Read the model definition and answer for the solid it produces. Units are mm, in the model's axes. Give positions to 0.01 mm unless a question says otherwise; leave off trailing zeros. Order: outer loops, then holes, each group sorted by start corner. A loop starts at its lowest first (then second) coordinate and runs counter-clockwise, first axis right, second up. Notation, with made-up numbers: (-30.5, 3.5) - (-19.5, 3.5) arc R29 cw to (-19.5, 36.5) - close; hole circle Ø8 at (83, 54). An arc over 180 degrees is marked (long way). Write each question's results on one line, items separated by ' | '.
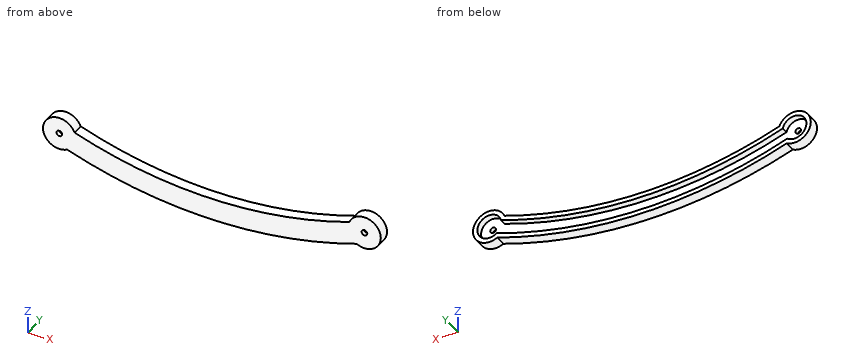
from build123d import *

# Parameters (mm, degrees)
DODANIE_WYCI_GNI_CIE2_DEPTH  = 5
SKORUPA2_START               = 2
SKORUPA2_DEPTH               = 3
SZKIC5_W                     = 1.3
SZKIC5_H                     = 2.001
OTW_R_POD_RUB_M22_AT_2_COUNT = 2
OTW_R_POD_RUB_M22_AT_2_PITCH = 140


# Read off the part's stored shape, not the designer's step: Skorupa2
with BuildPart() as part:
    # Szkic4 → Dodanie-wyciągnięcie2 (new body)
    with BuildSketch(Plane(origin=(0, 0, 0), x_dir=(1, 0, 0), z_dir=(0, 1, 0))):
        with BuildLine():
            ThreePointArc((3.578481933, 6.591241693), (-7.061624869, -2.526549863), (6.947544161, -2.825177894))
            ThreePointArc((6.947544161, -2.825177894), (70, 7.650060048), (133.052455839, -2.825177894))
            ThreePointArc((133.052455839, -2.825177894), (147.061624869, -2.526549863), (136.421518067, 6.591241693))
            ThreePointArc((136.421518067, 6.591241693), (70, 17.650060048), (3.578481933, 6.591241693))
        make_face()
    extrude(amount=DODANIE_WYCI_GNI_CIE2_DEPTH)

    # Skorupa2 outline → Skorupa2 (cut)
    with BuildSketch(Plane(origin=(0, 0, 0), x_dir=(1, 0, 0), z_dir=(0, 1, 0)).offset(SKORUPA2_START)):
        with BuildLine():
            ThreePointArc((3.318777837, 4.385853813), (-5.173966338, -1.865495198), (5.353998671, -1.258847978))
            ThreePointArc((5.353998671, -1.258847978), (70, 9.650060048), (134.646001329, -1.258847978))
            ThreePointArc((134.646001329, -1.258847978), (145.173966338, -1.865495198), (136.681222163, 4.385853813))
            ThreePointArc((136.681222163, 4.385853813), (70, 15.650060048), (3.318777837, 4.385853813))
        make_face()
    extrude(amount=SKORUPA2_DEPTH, mode=Mode.SUBTRACT)

    # Szkic5 → Otwór pod śrubę M22 (revolve, cut)
    with BuildSketch(Plane(origin=(0, 2, 0), x_dir=(0, 0, 1), z_dir=(1, 0, 0))):
        with Locations((0.65, 1.0005)):
            Rectangle(SZKIC5_W, SZKIC5_H)
    otw_r_pod_rub_m22 = revolve(axis=Axis((0, 8.35, 0), (0, -1, 0)), mode=Mode.SUBTRACT)

    # Otwór pod śrubę M22 at 2: Otwór pod śrubę M22 ×2
    with Locations(*[(i * OTW_R_POD_RUB_M22_AT_2_PITCH, 0, 0) for i in range(1, OTW_R_POD_RUB_M22_AT_2_COUNT)]):
        add(otw_r_pod_rub_m22, mode=Mode.SUBTRACT)


solid = part.part
(1) Section B-B (y = 3.7) is taken. Give the vertices of the cut face in (x, z), plus the area to 3 significant figures.
Conclusion:
outline: (3.58, -6.59) arc R205 ccw to (136.42, -6.59) arc R7.5 ccw (long way) to (133.05, 2.83) arc R195 cw to (6.95, 2.83) arc R7.5 ccw (long way) to start; hole (3.32, -4.39) arc R203 ccw to (136.68, -4.39) arc R5.5 ccw (long way) to (134.65, 1.26) arc R197 cw to (5.35, 1.26) arc R5.5 ccw (long way) to start | area: 660 mm^2
(2) Section A-A (x = 140) is taken. Give the vertices of the cut face in (y, z), plus the area to 3 significant figures.
Conclusion:
outline: (0, -7.5) - (5, -7.5) - (5, -5.5) - (2, -5.5) - (2, -1.3) - (0, -1.3) - close; (0, 1.3) - (2, 1.3) - (2, 5.5) - (5, 5.5) - (5, 7.5) - (0, 7.5) - close | area: 36.8 mm^2
(3) Consider probe 1 along Z at (x, y) = (140, 1.65); probe 2 along Z at (x, y) = (140, 4.35); probe 3 along X at (y, z) = (4.2, 4.75). Determine where each line is inside the solid, lowest interval first. Write a range as [from, to].
Conclusion:
probe 1: [-7.5, -1.3], [1.3, 7.5] | probe 2: [-7.5, -5.5], [5.5, 7.5] | probe 3: [-5.8, -2.77], [2.77, 5.8], [134.2, 137.23], [142.77, 145.8]
(4) This flat-tipped pin is pushed along its axis until it touches: pin 1 (9 mm diameter, centred on x = 140, z = 0, fed in from +Y). Where does it stop, or does it pass through?
Conclusion:
pin 1: y = 2
(5) Section C-C (z = 0) is taken. Give the vertices of the cut face in (x, y), plus the area to 3 significant figures.
Conclusion:
outline: (-7.5, 0) - (-1.3, 0) - (-1.3, 2) - (-5.5, 2) - (-5.5, 5) - (-7.5, 5) - close; (1.3, 0) - (15.92, 0) - (15.92, 5) - (9.1, 5) - (9.1, 2) - (1.3, 2) - close; (124.08, 0) - (138.7, 0) - (138.7, 2) - (130.9, 2) - (130.9, 5) - (124.08, 5) - close; (141.3, 0) - (147.5, 0) - (147.5, 5) - (145.5, 5) - (145.5, 2) - (141.3, 2) - close | area: 136 mm^2
(6) Section D-D (x = 101) is taken. Give the vertices of the cut face in (y, z).
Conclusion:
outline: (0, -15.29) - (5, -15.29) - (5, -13.27) - (2, -13.27) - (2, -7.2) - (5, -7.2) - (5, -5.17) - (0, -5.17) - close
